```python
from build123d import *

# Parameters (mm, degrees)
BOSS_EXTRUDE1_DEPTH                        = 3
SKETCH3_R                                  = 1.75
CUT_EXTRUDE1_DEPTH                         = 124.780046857
MIRROR1_AT_THE_SECOND_PLANE_COPY_1_SKETC_R = 1.75
MIRROR1_AT_THE_SECOND_PLANE_COPY_1_DEPTH   = 124.780046857


with BuildPart() as part:
    # Sketch1 → Boss-Extrude1 (new body)
    with BuildSketch(Plane.XY):
        with BuildLine():
            Line((-30, 57.196411114), (30, 57.196411114))
            Line((30, 57.196411114), (30, 82.196411114))
            ThreePointArc((30, 82.196411114), (0, -87.5), (-30, 82.196411114))
            Line((-30, 82.196411114), (-30, 57.196411114))
        make_face()
    extrude(amount=-BOSS_EXTRUDE1_DEPTH)

    # Sketch3 → Cut-Extrude1 (cut, through all)
    with BuildSketch(Plane.XY):
        with BuildLine():
            Line((-61.559070668, 36.810333327), (-47.416935045, 22.668197703))
            Line((-47.416935045, 22.668197703), (-22.668197703, 47.416935045))
            Line((-22.668197703, 47.416935045), (-36.810333327, 61.559070668))
            Line((-36.810333327, 61.559070668), (-33.274799421, 65.094604574))
            Line((-33.274799421, 65.094604574), (-43.881401139, 75.701206292))
            ThreePointArc((-43.881401139, 75.701206292), (-61.871843354, 61.871843354), (-75.701206292, 43.881401139))
            Line((-75.701206292, 43.881401139), (-65.094604574, 33.274799421))
            Line((-65.094604574, 33.274799421), (-61.559070668, 36.810333327))
        make_face()
        with Locations((-60.851963887, 20.54687736)):
            Circle(SKETCH3_R)
        with Locations((-20.54687736, 60.851963887)):
            Circle(SKETCH3_R)
    cut_extrude1 = extrude(amount=-CUT_EXTRUDE1_DEPTH, mode=Mode.SUBTRACT)

    # Mirror1: Cut-Extrude1 across plane
    add(cut_extrude1.mirror(Plane(origin=(0, 0, 0), x_dir=(0, 0, 1), z_dir=(1, 0, 0))), mode=Mode.SUBTRACT)

    # Mirror1 at the second plane: Cut-Extrude1 across plane
    add(cut_extrude1.mirror(Plane.ZX), mode=Mode.SUBTRACT)

    # Mirror1 at the second plane copy 1 sketc → Mirror1 at the second plane copy 1 (cut, through all)
    with BuildSketch(Plane(origin=(0, 0, 0), x_dir=(-1, 0, 0), z_dir=(0, 0, 1))):
        with BuildLine():
            Line((-61.559070668, 36.810333327), (-47.416935045, 22.668197703))
            Line((-47.416935045, 22.668197703), (-22.668197703, 47.416935045))
            Line((-22.668197703, 47.416935045), (-36.810333327, 61.559070668))
            Line((-36.810333327, 61.559070668), (-33.274799421, 65.094604574))
            Line((-33.274799421, 65.094604574), (-43.881401139, 75.701206292))
            ThreePointArc((-43.881401139, 75.701206292), (-61.871843354, 61.871843354), (-75.701206292, 43.881401139))
            Line((-75.701206292, 43.881401139), (-65.094604574, 33.274799421))
            Line((-65.094604574, 33.274799421), (-61.559070668, 36.810333327))
        make_face()
        with Locations((-60.851963887, 20.54687736)):
            Circle(MIRROR1_AT_THE_SECOND_PLANE_COPY_1_SKETC_R)
        with Locations((-20.54687736, 60.851963887)):
            Circle(MIRROR1_AT_THE_SECOND_PLANE_COPY_1_SKETC_R)
    extrude(amount=-MIRROR1_AT_THE_SECOND_PLANE_COPY_1_DEPTH, mode=Mode.SUBTRACT)


solid = part.part
```
CAD build for the part. Positions are in the model's coordinates, mm. A direction names the side the tool comes from. Coordinates: 2 decimals unless noted, no trailing zeros. Order: outer loops, then holes, each group sorted by start corner. A loop starts at its lowest first (then second) coordinate and runs counter-clockwise, first axis right, second up. Notation, with made-up numbers: (73, 88.25) - (110, 88.25) arc R31 cw to (110, 112.25) - close; hole circle Ø11 at (18, -4.75). An arc over 180 degrees is marked (long way). Use a Markdown table: item, result. Add a question column.
(1) Drill centre lines: line 1 along X through (y, z) = (42, -1.2); line 2 along X through (y, z) = (-42.5, -2.35); line 3 along Y through (x, z) = (-27, -1.1). Where is each one in solid material? Low to high. Write a range as [from, to].
(2) Which spindle directions (+Z, -Z, +X, -X, +Y, -Y) get a long thin tool onto all of the face, cutting with end or side? Do faces 1 (the face through (29.64, -54.39, -1.48)), 2 (the face through (-70.47, -38.65, -1.48)), 3 (the face through (-70.47, 38.65, -1.48)). Say none if no direction does.
(3) Saw through at A-A (y = -28). Give the cut face in (x, z).
(4) Saw through at D-D (x = -16). Give the cut face in (y, z).
(5) Saw through at B-B (x = 27.5). Give the cut face in (y, z), then the cut area to 3 significant figures.
(6) Pull direction Y, two halves, no side cores. Call faces 4 (the face through (-37.2, 79.2, -1.5)), 5 (the face through (0.644, -87.498, -1.479)), 6 (the face through (29.64, 54.39, -1.48)): +Y half, -Y half, draft (parallel to the pull), parting line (faces both ways), or undercut.
(7) Saw through at C-C (z = -1.4). Count the separate pieces of the cut face and the enclosed holes in it, then the cut area to 3 significant figures.
(8) Flat gauge pins, fed straight in: pin 1 (1.5 mm diameter, centred on x = -2, z = -1, fed in from +Y); pin 2 (4.5 mm diameter, centred on x = -60.85, y = 20.55, fed in from +Z); pin 3 (1.5 mm diameter, centred on y = 72, z = -1, fed in from -X); pin 4 (1 mm diameter, centred on y = 53.5, z = -2, fed in from +X). Where does each tip first touch, or does it go through?
Solved:
| question | item | result |
|---|---|---|
| 1 | line 1 | x = [-76.76, -73.82], [-28.09, 28.09], [73.82, 76.76] |
| 1 | line 2 | x = [-76.49, -74.32], [-27.59, 27.59], [74.32, 76.49] |
| 1 | line 3 | y = [-83.23, -51.75], [-43.09, 43.09], [51.75, 57.2] |
| 2 | face 1 | +Z, -Z, +X |
| 2 | face 2 | +Z, -Z, -Y |
| 2 | face 3 | +Z, -Z, +Y |
| 3 | outline | (-82.9, -3) - (-52.75, -3) - (-52.75, 0) - (-82.9, 0) - close; (-42.09, -3) - (42.09, -3) - (42.09, 0) - (-42.09, 0) - close; (52.75, -3) - (82.9, -3) - (82.9, 0) - (52.75, 0) - close |
| 4 | outline | (-86.02, -3) - (57.2, -3) - (57.2, 0) - (-86.02, 0) - close |
| 5 | outline | (-83.07, -3) - (-52.25, -3) - (-52.25, 0) - (-83.07, 0) - close; (-42.59, -3) - (42.59, -3) - (42.59, 0) - (-42.59, 0) - close; (52.25, -3) - (57.2, -3) - (57.2, 0) - (52.25, 0) - close |
| 5 | area | 363 mm² |
| 6 | face 4 | +Y half |
| 6 | face 5 | -Y half |
| 6 | face 6 | undercut |
| 7 | separate pieces | 1 |
| 7 | enclosed holes | 6 |
| 7 | area | 16,400 mm² |
| 8 | pin 1 | stops at y = 57.2 |
| 8 | pin 2 | stops at z = 0 |
| 8 | pin 3 | stops at x = -40.93 |
| 8 | pin 4 | stops at x = 29.25 |
